```python
from build123d import *

# Parameters (mm, degrees)
F1_R     = 1.65
F2_DEPTH = 3.2
F2_TAPER = -3
F0_R     = 1.65
F3_DEPTH = 3.2
F5_R     = 5
F6_DEPTH = 3.3
F4_R     = 1.65
F7_DEPTH = 3.3
F8_R     = 1.65
F9_DEPTH = 3.2


with BuildPart() as f2:
    # F1 (on Top) → F2 (new body)
    with BuildSketch(Plane.XY):
        with BuildLine():
            ThreePointArc((-5, 0), (0, -5), (5, 0))
            ThreePointArc((5, 0), (0, 5), (-5, 0))
        make_face()
        Circle(F1_R, mode=Mode.SUBTRACT)
        with BuildLine():
            Line((5, -30), (5, 0))
            ThreePointArc((5, 0), (0, -5), (-5, 0))
            Line((-5, 0), (-5, -30))
            ThreePointArc((-5, -30), (0, -25), (5, -30))
        make_face()
        with BuildLine():
            ThreePointArc((-5, -30), (0, -35), (5, -30))
            ThreePointArc((5, -30), (0, -25), (-5, -30))
        make_face()
    extrude(amount=F2_DEPTH, taper=F2_TAPER)

    # F0 (on Top) → F3 (cut)
    with BuildSketch(Plane.XY):
        Circle(F0_R)
    extrude(amount=F3_DEPTH, mode=Mode.SUBTRACT)

    # F5 (on Top) → F6 (join)
    with BuildSketch(Plane.XY):
        Circle(F5_R)
    extrude(amount=-F6_DEPTH)

    # F4 (on Top) → F7 (cut)
    with BuildSketch(Plane.XY):
        Circle(F4_R)
    extrude(amount=-F7_DEPTH, mode=Mode.SUBTRACT)

    # F8 (on Top) → F9 (cut)
    with BuildSketch(Plane.XY):
        with Locations((0, -30)):
            Circle(F8_R)
    extrude(amount=F9_DEPTH, mode=Mode.SUBTRACT)


solid = f2.part
```
CAD build for the part. Positions are in the model's coordinates, mm. Coordinates: 2 decimals unless noted, no trailing zeros. Order: outer loops, then holes, each group sorted by start corner. A loop starts at its lowest first (then second) coordinate and runs counter-clockwise, first axis right, second up. Notation, with made-up numbers: (78.5, 29.25) - (90.5, 29.25) arc R20 ccw to (90.5, 42.25) - close; hole circle Ø2 at (-39, 33). An arc over 180 degrees is marked (long way). Use a Markdown table: item, result. Add a question column.
(1) Drill centre lines: line 1 along Y through (x, z) = (0, -2.4); line 2 along Y through (x, z) = (0.5, 1.5); line 3 along Y through (x, z) = (0, 0.7). Where is each one in solid material? Low to high. Write a range as [from, to].
(2) Pull direction Y, two halves, no side cores. Call faces 1 (the face through (0.112, 5.084, 1.622)), 2 (the face through (-0.215, -28.364, 1.578)), 3 (the face through (0, -15, 3.2)), 4 (the face through (-1.08, -4.88, -1.63)): +Y half, -Y half, draft (parallel to the pull), parting line (faces both ways), or undercut.
(3) Saw through at A-A (x = 0). Give the cut face in (y, z).
(4) Flat gauge pins, fed straight in: pin 1 (2 mm diameter, centred on x = 0, y = 0, fed in from -Z); pin 2 (2 mm diameter, centred on x = 2.5, z = 1, fed in from +Y); pin 3 (5.5 mm diameter, centred on x = 0, y = -30, fed in from -Z). Where does each tip first touch, or does it go through?
(5) Saw through at B-B (z = 0.5). Give the cut face in (x, y), then the cut area to 3 significant figures.
(6) Saw through at C-C (y = -18). Give the cut face in (x, z), then the cut area to 3 significant figures.
Solved:
| question | item | result |
|---|---|---|
| 1 | line 1 | y = [-5, -1.65], [1.65, 5] |
| 1 | line 2 | y = [-35.05, -31.57], [-28.43, -1.57], [1.57, 5.05] |
| 1 | line 3 | y = [-35.04, -31.65], [-28.35, -1.65], [1.65, 5.04] |
| 2 | face 1 | +Y half |
| 2 | face 2 | undercut |
| 2 | face 3 | draft |
| 2 | face 4 | parting line |
| 3 | outline | (-35.17, 3.2) - (-35, 0) - (-31.65, 0) - (-31.65, 3.2) - close; (-28.35, 0) - (-5, 0) - (-5, -3.3) - (-1.65, -3.3) - (-1.65, 3.2) - (-28.35, 3.2) - close; (1.65, -3.3) - (5, -3.3) - (5, 0) - (5.17, 3.2) - (1.65, 3.2) - close |
| 4 | pin 1 | passes through |
| 4 | pin 2 | stops at y = 4.83 |
| 4 | pin 3 | stops at z = 0 |
| 5 | outline | (-5.03, -30) arc R5.03 ccw to (5.03, -30) - (5.03, 0) arc R5.03 ccw to (-5.03, 0) - close; hole circle Ø3.3 at (0, -30); hole circle Ø3.3 at (0, 0) |
| 5 | area | 364 mm² |
| 6 | outline | (-5.17, 3.2) - (-5, 0) - (5, 0) - (5.17, 3.2) - close |
| 6 | area | 32.5 mm² |
